```python
from build123d import *

# Parameters (mm, degrees)
BOSS_EXTRUDE3_DEPTH = 152.4
CUT_EXTRUDE3_REACH  = 161.569
SKETCH7_R           = 6.35
SKETCH8_R           = 6.763254826
CUT_EXTRUDE4_DEPTH  = 162.893869557


with BuildPart() as part:
    # Sketch6 → Boss-Extrude3 (new body)
    with BuildSketch(Plane(origin=(0, 0, 0), x_dir=(0, 0, -1), z_dir=(1, 0, 0))):
        Polygon((-35.048704326, 0), (9.401295674, 0), (9.401295674, -31.75), (3.051295674, -31.75), (3.051295674, -6.35), (-28.698704326, -6.35), (-28.698704326, -31.75), (-35.048704326, -31.75), align=None)
    extrude(amount=BOSS_EXTRUDE3_DEPTH)

    # Sketch7 → Cut-Extrude3 (cut, up to next)
    with BuildSketch(Plane(origin=(0, 0, 0), x_dir=(1, 0, 0), z_dir=(0, 1, 0)), mode=Mode.PRIVATE) as cut_extrude3_sk1:
        with Locations(Location((76.2, -12.823704326, 0), (0, 0, 270))):
            Circle(SKETCH7_R)
    cut_extrude3_tool1 = extrude(cut_extrude3_sk1.sketch, amount=-CUT_EXTRUDE3_REACH, mode=Mode.PRIVATE) & part.part
    add(cut_extrude3_tool1.solids().sort_by_distance((76.2, 0, 12.823704))[0], mode=Mode.SUBTRACT)

    # Sketch8 → Cut-Extrude4 (cut, through all)
    with BuildSketch(Plane.XY.offset(35.048704326)):
        with Locations((12.7, -19.05)):
            Circle(SKETCH8_R)
        with Locations(Location((139.7, -19.05, 0), (0, 0, 180))):
            Circle(SKETCH8_R)
    extrude(amount=-CUT_EXTRUDE4_DEPTH, mode=Mode.SUBTRACT)


solid = part.part
```
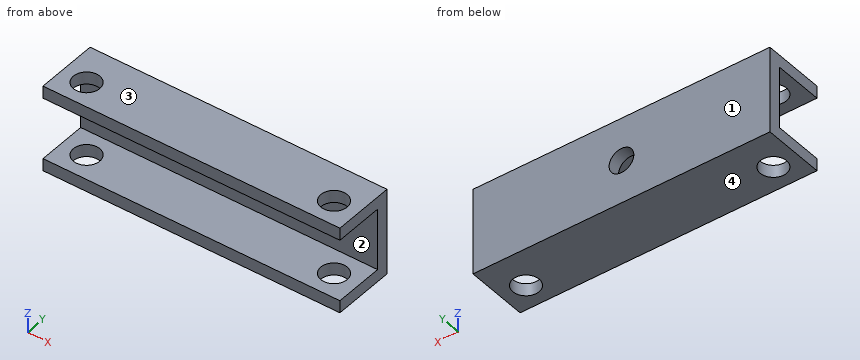
Build history of the part. All positions in model axes, mm. Face numbers are marked on the shaded views. Round coordinates to 2 decimals unless told otherwise and drop trailing zeros. Write each loop counter-clockwise with the first axis right and the second up, starting at its lowest first coordinate (ties: lowest second). Pieces come first, ordered by that corner, then holes. Notation, with made-up numbers: (74, 13) - (133, 13) arc R35 cw to (133, 46) - close; hole circle Ø7 at (81.5, 82.25). An arc over 180 degrees is marked (long way). Write each question's results on one line, items separated by ' | '. Start each with the question number.
Item 1: Drop a flat-ended pin along its axis: P1, Ø8, axis at y = -11, z = 15.5, coming from the -X side. Give the stop position or say it passes through.
Item 2: Saw through at D-D (x = 12.7). Write the cut outline in (y, z).
Item 3: Saw through at B-B (x = 76.2). Write the cut outline in (y, z), and give its area (3 significant figures).
Item 4: Mould opens along Z. For the marked faces 1, 2, 3 and 4 say: pulls with the +Z half, pulls with the -Z half, needs draft (parallel to the pull), parting line crosses it, or undercut.
Item 5: Saw through at C-C (y = -19.05). Write the cut outline in (x, z).
Item 6: Wall check: L1, parallel to Z at x = 13.5, y = -27; L2, parallel to X at y = -19, z = 32; L3, parallel to Y at x = 139.7, z = -8. Give the ranges that are in metal, low to high. Write a range as [from, to].
Item 7: Saw through at A-A (y = -28.5). Write the cut outline in (x, z), and give its area (3 significant figures).
Results are:
1) P1: passes through
2) outline: (-31.75, -9.4) - (-25.81, -9.4) - (-25.81, -3.05) - (-31.75, -3.05) - close; (-31.75, 28.7) - (-25.81, 28.7) - (-25.81, 35.05) - (-31.75, 35.05) - close; (-12.29, -9.4) - (0, -9.4) - (0, 35.05) - (-12.29, 35.05) - (-12.29, 28.7) - (-6.35, 28.7) - (-6.35, -3.05) - (-12.29, -3.05) - close
3) outline: (-31.75, -9.4) - (0, -9.4) - (0, 6.47) - (-6.35, 6.47) - (-6.35, -3.05) - (-31.75, -3.05) - close; (-31.75, 28.7) - (-6.35, 28.7) - (-6.35, 19.17) - (0, 19.17) - (0, 35.05) - (-31.75, 35.05) - close | area: 524 mm²
4) face 1: needs draft | face 2: undercut | face 3: pulls with the +Z half | face 4: pulls with the -Z half
5) outline: (0, -9.4) - (5.94, -9.4) - (5.94, -3.05) - (0, -3.05) - close; (0, 28.7) - (5.94, 28.7) - (5.94, 35.05) - (0, 35.05) - close; (19.46, -9.4) - (132.94, -9.4) - (132.94, -3.05) - (19.46, -3.05) - close; (19.46, 28.7) - (132.94, 28.7) - (132.94, 35.05) - (19.46, 35.05) - close; (146.46, -9.4) - (152.4, -9.4) - (152.4, -3.05) - (146.46, -3.05) - close; (146.46, 28.7) - (152.4, 28.7) - (152.4, 35.05) - (146.46, 35.05) - close
6) L1: z = [-9.4, -3.05], [28.7, 35.05] | L2: x = [0, 5.94], [19.46, 132.94], [146.46, 152.4] | L3: y = [-31.75, -25.81], [-12.29, 0]
7) outline: (0, -9.4) - (152.4, -9.4) - (152.4, -3.05) - (0, -3.05) - close; (0, 28.7) - (152.4, 28.7) - (152.4, 35.05) - (0, 35.05) - close | area: 1,940 mm²
